Could you check a few things on this model? Use its own coordinates, in mm. Give positions to 0.01 mm unless a question says otherwise; leave off trailing zeros. Loops run counter-clockwise (first coordinate to the right, second up) from the corner with the lowest first, then second, coordinate; pieces in that order, holes last.
1. Imagine slicing it at A-A (z = -24). List the corners of the cut face in (x, y) for me.
2. Imagine slicing it at B-B (z = 3.5). List the corners of the cut face in (x, y) for me.
3. I need wall thicknesses on line 1 along Y through (x, z) = (114.5, -25); line 2 along Y through (x, z) = (124.25, -25.5); line 3 along X through (y, z) = (119, -22). Which ranges of each line are inside material? Lowest first, please.
4. For P1, Ø1, axis at y = 122.5, z = -14, coming from the -X side; P2, Ø8, axis at y = 114.5, z = -22, coming from the -X side; P3, Ø10, axis at y = 133.5, z = -27.5, coming from the +X side; P4, Ø10, axis at y = 123, z = -28.5, coming from the -X side, each with a flat end and sliding along its axis, tell me the tip position at first contact or that it passes through.
```python
from build123d import *

# Parameters (mm, degrees)
BOSS_EXTRUDE1_DEPTH      = 2.54
BOSS_EXTRUDE1_DEPTH_BACK = 27.94
SKETCH1_R                = 12.7
DOME1_FACE_RADIUS        = 12.7
DOME1_HEIGHT             = 5.08
DOME2_FACE_RADIUS        = 12.7
DOME2_HEIGHT             = 5.08


with BuildPart() as part:
    # Sketch1 → Boss-Extrude1 (new, two sides: drawn at the far end of the back side and taken through both)
    with BuildSketch(Plane.XY.offset(-BOSS_EXTRUDE1_DEPTH_BACK)):
        with Locations((114.42340137, 123.880750733)):
            Circle(SKETCH1_R)
    extrude(amount=BOSS_EXTRUDE1_DEPTH + BOSS_EXTRUDE1_DEPTH_BACK)

    # Dome1: an elliptical dome of height H over a round flat face of radius A is half a spheroid: the quarter ellipse of half axes A and H revolved about the face's axis
    with BuildSketch(Plane((114.42340137, 123.880750733, -27.94), x_dir=(0, -1, 0), z_dir=(1, 0, 0)), mode=Mode.PRIVATE) as dome1_quarter:
        Ellipse(DOME1_FACE_RADIUS, DOME1_HEIGHT)
        Rectangle(DOME1_FACE_RADIUS, DOME1_HEIGHT, align=(Align.MIN, Align.MIN), mode=Mode.INTERSECT)
    revolve(dome1_quarter.sketch, axis=Axis((114.42340137, 123.880750733, -27.94), (0, 0, -1)))

    # Dome2: a dome of height H over a round flat face of radius A is a cap of a sphere of radius (A * A + H * H) / (2 * H)
    dome2_r = (DOME2_FACE_RADIUS * DOME2_FACE_RADIUS + DOME2_HEIGHT * DOME2_HEIGHT) / (2 * DOME2_HEIGHT)
    dome2_base = Plane((114.42340137, 123.880750733, 2.54), z_dir=(0, 0, 1))
    with Locations(dome2_base.offset(DOME2_HEIGHT - dome2_r)):
        dome2_ball = Sphere(dome2_r, mode=Mode.PRIVATE)
    add(split(dome2_ball, bisect_by=dome2_base, keep=Keep.TOP, mode=Mode.PRIVATE))


solid = part.part
```
Derived:
1. outline: circle Ø25.4 at (114.42, 123.88)
2. outline: circle Ø23.22 at (114.42, 123.88)
3. line 1: y = 111.18 to 136.58
3. line 2: y = 115.84 to 131.93
3. line 3: x = 102.7 to 126.15
4. P1: stops at x = 101.75
4. P2: stops at x = 102.92
4. P3: stops at x = 126.25
4. P4: stops at x = 101.72
